Part model, mm, in its own coordinate system. A direction names the side the tool comes from. Give positions to 0.01 mm unless a question says otherwise; leave off trailing zeros. Loops run counter-clockwise (first coordinate to the right, second up) from the corner with the lowest first, then second, coordinate; pieces in that order, holes last. Notation, with made-up numbers: (62.25, 51) -> (66.25, 51) arc R27 ccw to (66.25, 83) -> close; hole circle Ø9 at (39.5, 61.25). An arc over 180 degrees is marked (long way). One line per question, with ' | ' between items.
```python
from build123d import *

# Parameters (mm, degrees)
SKETCH1_W           = 84
SKETCH1_H           = 180
BOSS_EXTRUDE1_DEPTH = 7
SKETCH2_R           = 1.775
CUT_EXTRUDE1_DEPTH  = 103.960355362
SKETCH3_R           = 3.05
CUT_EXTRUDE2_DEPTH  = 4
SKETCH5_W           = 12
SKETCH5_H           = 12
SKETCH5_W_2         = 14
BOSS_EXTRUDE2_DEPTH = 14
SKETCH6_R           = 1.775
CUT_EXTRUDE3_DEPTH  = 105.846720389
SKETCH7_R           = 2
CUT_EXTRUDE4_DEPTH  = 105.846720389
SKETCH8_R           = 1.775
CUT_EXTRUDE5_DEPTH  = 105.846720389


with BuildPart() as part:
    # Sketch1 → Boss-Extrude1 (new body)
    with BuildSketch(Plane(origin=(0, 0, 0), x_dir=(1, 0, 0), z_dir=(0, 1, 0))):
        with Locations((-5.498242658, 1.081017345)):
            Rectangle(SKETCH1_W, SKETCH1_H)
    extrude(amount=BOSS_EXTRUDE1_DEPTH)

    # Sketch2 → Cut-Extrude1 (cut, through all)
    with BuildSketch(Plane(origin=(0, 7, 0), x_dir=(1, 0, 0), z_dir=(0, 1, 0))):
        with Locations(Location((-40.498242658, 1.081017345, 0), (0, 0, 270))):
            Circle(SKETCH2_R)
        with Locations(Location((-5.498242658, -33.918982655, 0), (0, 0, 270))):
            Circle(SKETCH2_R)
        with Locations(Location((29.501757342, 1.081017345, 0), (0, 0, 270))):
            Circle(SKETCH2_R)
        with Locations(Location((-5.498242658, 36.081017345, 0), (0, 0, 270))):
            Circle(SKETCH2_R)
    extrude(amount=-CUT_EXTRUDE1_DEPTH, mode=Mode.SUBTRACT)

    # Sketch3 → Cut-Extrude2 (cut)
    with BuildSketch(Plane(origin=(0, 7, 0), x_dir=(1, 0, 0), z_dir=(0, 1, 0))):
        with Locations(Location((-40.498242658, 1.081017345, 0), (0, 0, 270))):
            Circle(SKETCH3_R)
        with Locations(Location((-5.498242658, -33.918982655, 0), (0, 0, 270))):
            Circle(SKETCH3_R)
        with Locations(Location((-5.498242658, 36.081017345, 0), (0, 0, 270))):
            Circle(SKETCH3_R)
        with Locations(Location((29.501757342, 1.081017345, 0), (0, 0, 270))):
            Circle(SKETCH3_R)
    extrude(amount=-CUT_EXTRUDE2_DEPTH, mode=Mode.SUBTRACT)

    # Sketch5 → Boss-Extrude2 (add)
    with BuildSketch(Plane(origin=(0, 0, 0), x_dir=(-1, 0, 0), z_dir=(0, -1, 0))):
        with Locations((5.498242658, -33.918982655)):
            Rectangle(SKETCH5_W, SKETCH5_H)
        with Locations((40.498242658, 1.081017345)):
            Rectangle(SKETCH5_W_2, SKETCH5_H)
        with Locations((5.498242658, 36.081017345)):
            Rectangle(SKETCH5_W, SKETCH5_H)
        with Locations((-29.501757342, 1.081017345)):
            Rectangle(SKETCH5_W_2, SKETCH5_H)
    extrude(amount=BOSS_EXTRUDE2_DEPTH)

    # Sketch6 → Cut-Extrude3 (cut, through all)
    with BuildSketch(Plane(origin=(0, 7, 0), x_dir=(1, 0, 0), z_dir=(0, 1, 0))):
        with Locations(Location((-40.498242658, 1.081017345, 0), (0, 0, 270))):
            Circle(SKETCH6_R)
        with Locations(Location((29.501757342, 1.081017345, 0), (0, 0, 270))):
            Circle(SKETCH6_R)
        with Locations(Location((-5.498242658, -33.918982655, 0), (0, 0, 270))):
            Circle(SKETCH6_R)
        with Locations(Location((-5.498242658, 36.081017345, 0), (0, 0, 270))):
            Circle(SKETCH6_R)
    extrude(amount=-CUT_EXTRUDE3_DEPTH, mode=Mode.SUBTRACT)

    # Sketch7 → Cut-Extrude4 (cut, through all)
    with BuildSketch(Plane(origin=(0, 7, 0), x_dir=(1, 0, 0), z_dir=(0, 1, 0))):
        with Locations(Location((-35.998242658, -63.918982655, 0), (0, 0, 270))):
            Circle(SKETCH7_R)
        with Locations(Location((-35.998242658, -11.418982655, 0), (0, 0, 270))):
            Circle(SKETCH7_R)
        with Locations(Location((-35.998242658, 41.081017345, 0), (0, 0, 270))):
            Circle(SKETCH7_R)
        with Locations(Location((25.001757342, -63.918982655, 0), (0, 0, 270))):
            Circle(SKETCH7_R)
        with Locations(Location((25.001757342, -11.418982655, 0), (0, 0, 270))):
            Circle(SKETCH7_R)
        with Locations(Location((25.001757342, 41.081017345, 0), (0, 0, 270))):
            Circle(SKETCH7_R)
    extrude(amount=-CUT_EXTRUDE4_DEPTH, mode=Mode.SUBTRACT)

    # Sketch8 → Cut-Extrude5 (cut, through all)
    with BuildSketch(Plane(origin=(0, 7, 0), x_dir=(1, 0, 0), z_dir=(0, 1, 0))):
        with Locations(Location((-39.998242658, -81.418982655, 0), (0, 0, 270))):
            Circle(SKETCH8_R)
        with Locations(Location((-39.998242658, 83.581017345, 0), (0, 0, 270))):
            Circle(SKETCH8_R)
        with Locations(Location((29.001757342, 83.581017345, 0), (0, 0, 270))):
            Circle(SKETCH8_R)
        with Locations(Location((29.001757342, -81.418982655, 0), (0, 0, 270))):
            Circle(SKETCH8_R)
    extrude(amount=-CUT_EXTRUDE5_DEPTH, mode=Mode.SUBTRACT)


solid = part.part
```
1) Pull direction Z, two halves, no side cores. Call faces 5 (the cylindrical face through (27.77, -5.38, -1.47)), 6 (the flat face through (30, -7, -7.081)), 7 (the flat face through (-11.498, -7, 34)): pulls with the +Z half, pulls with the -Z half, needs draft (parallel to the pull), parting line crosses it, or undercut.
Found:
face 5: undercut | face 6: pulls with the -Z half | face 7: needs draft
2) Drill centre lines: line 1 (Z direction, x = 25, y = 0.5); line 2 (Y direction, x = -22, z = 6); line 3 (Z direction, x = -36.5, y = 1.5). Where is each one in solid material? Low to high.
Found:
line 1: -91.08 to -43.08, -39.08 to 9.42, 13.42 to 61.92, 65.92 to 88.92 | line 2: 0 to 7 | line 3: -91.08 to -43.02, -39.14 to 9.48, 13.36 to 61.98, 65.86 to 88.92
3) Pin check, flat tips, straight feed: P1, Ø3.5, axis at y = -9.5, z = 33.5, coming from the -X side; P2, Ø1.8, axis at x = -6.5, z = 32.5, coming from the +Y side; P3, Ø5.5, axis at x = 29, z = -83.58, coming from the -Y side. Stop position of each tip, or through.
Found:
P1: x = -11.5 | P2: y = 3 | P3: y = 0
4) Tool access for faces 1 (the flat face through (-6, 0, -2)), 2 (the flat face through (-40, -7, 4.919)), 3 (the cylindrical face through (-43.476, 5.028, -1.742)), 4 (the flat face through (-11.498, -7, -36)): list every direction of +Z, -Z, +X, -X, +Y, -Y with a clear straight run to the whole face (end or side of a thin tool).
Found:
face 1: -Y | face 2: +Z, +X, -X, -Y | face 3: +Y | face 4: +Z, -Z, -X, -Y
5) Saw through at C-C (x = 4). Give the cut face in (y, z).
Found:
outline: (0, -91.08) -> (7, -91.08) -> (7, 88.92) -> (0, 88.92) -> close
6) Saw through at A-A (y = -4.5). Give the cut face in (x, z) (3 decimals), and give its area (3 significant figures).
Found:
outline: (-47.498, -7.081) -> (-33.498, -7.081) -> (-33.498, 4.919) -> (-47.498, 4.919) -> close; (-11.498, -42.081) -> (0.502, -42.081) -> (0.502, -30.081) -> (-11.498, -30.081) -> close; (-11.498, 27.919) -> (0.502, 27.919) -> (0.502, 39.919) -> (-11.498, 39.919) -> close; (22.502, -7.081) -> (36.502, -7.081) -> (36.502, 4.919) -> (22.502, 4.919) -> close; hole circle Ø3.55 at (-40.498, -1.081); hole circle Ø3.55 at (-5.498, -36.081); hole circle Ø3.55 at (-5.498, 33.919); hole circle Ø3.55 at (29.502, -1.081) | area: 584 mm2
7) Saw through at B-B (z = 42). Give the cut face in (x, y), and give its area (3 significant figures).
Found:
outline: (-47.5, 0) -> (36.5, 0) -> (36.5, 7) -> (-47.5, 7) -> close | area: 588 mm2
